```python
from build123d import *

# Parameters (mm, degrees)
SKETCH1_R           = 39.3
BOSS_EXTRUDE1_DEPTH = 21.4
FILLET1_R           = 1.5
SKETCH2_R           = 4
CUT_EXTRUDE1_DEPTH  = 50


with BuildPart() as part:
    # Sketch1 → Boss-Extrude1 (new body)
    with BuildSketch(Plane(origin=(0, 0, 0), x_dir=(1, 0, 0), z_dir=(0, 1, 0))):
        Circle(SKETCH1_R)
    extrude(amount=BOSS_EXTRUDE1_DEPTH)

    # Fillet1
    fillet1_edges = [part.edges().sort_by_distance(p)[0] for p in [
        (-39.3, 21.4, 0),
    ]]
    fillet(fillet1_edges, radius=FILLET1_R)

    # Sketch2 → Cut-Extrude1 (cut)
    with BuildSketch(Plane.XY.offset(39.3)):
        with Locations((-20, 9.95)):
            Circle(SKETCH2_R)
        with Locations((20, 9.95)):
            Circle(SKETCH2_R)
    extrude(amount=-CUT_EXTRUDE1_DEPTH, mode=Mode.SUBTRACT)


solid = part.part
```
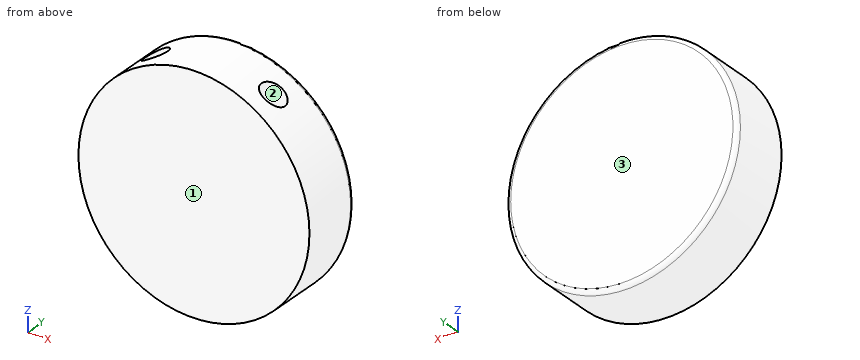
Can you work these out from the model? Positions are in its coordinate system, mm. Face numbers are marked on the shaded views. Coordinates: 2 decimals unless noted, no trailing zeros. Write each loop counter-clockwise with the first axis right and the second up, starting at its lowest first coordinate (ties: lowest second). Pieces come first, ordered by that corner, then holes. Notation, with made-up numbers: M 33,-11 L 77,-11 A14 cw 77,-1 Z; hole C 39.25,-24 d6. An arc over 180 degrees is marked long. Write item = value, one per line. Start each with the question number.
Q1. I'm going to push flat-ended pins straight in: pin 1 (4 mm diameter, centred on y = 8, z = 6, fed in from -X); pin 2 (6 mm diameter, centred on x = -26.5, y = 17.5, fed in from -Z); pin 3 (4 mm diameter, centred on x = -20, y = 10, fed in from +Z). Where does each tip first touch, or does it pass through?
Q2. If we section it at A-A, the plane z = 0: Write out the boundary of the cut face in (x, y).
Q3. If I drill on L1, parallel to Y at x = 20, z = 18; L2, parallel to X at y = 9.95, z = 0.5; L3, parallel to X at y = 9.95, z = 3, over which ranges is the centre line in solid material (lowest first)? Write a range as [from, to].
Q4. If we section it at B-B, the plane y = 17.75: Write out the boundary of the cut face in (x, z).
Q5. If we section it at D-D, the plane y = 9.95: Write out the boundary of the cut face in (x, z), then the cut area to 3 significant figures.
Q6. If we section it at C-C, the plane z = -8: State how many separate pieces and enclosed holes the cut face has, then the cut area to 3 significant figures.
Q7. Thinking about a two-plate mould opening in Y: for the marked faces 1, 2 and 3, which applies, released by +Y, released by -Y, zero draft, split by the parting line, or undercut?
Check sheet entries:
q1.pin_1 = -39.1
q1.pin_2 = -31.5
q1.pin_3 = -10.7
q2.outline = M -39.3,0 L 39.3,0 L 39.3,19.9 A1.5 ccw 37.8,21.4 L -37.8,21.4 A1.5 ccw -39.3,19.9 Z; hole C -20,9.95 d8; hole C 20,9.95 d8
q3.L1 = [0, 5.95], [13.95, 21.4]
q3.L2 = [-39.3, -24], [-16, 16], [24, 39.3]
q3.L3 = [-39.19, -24], [-16, 16], [24, 39.19]
q4.outline = C 0,0 d78.6
q5.outline = M -24,-10.7 L -24,31.12 A39.3 ccw long 24,31.12 L 24,-10.7 L 16,-10.7 L 16,35.9 A39.3 ccw -16,35.9 L -16,-10.7 Z
q5.area = 4,140 mm²
q6.separate_pieces = 1
q6.enclosed_holes = 2
q6.area = 1,550 mm²
q7.face_1 = released by -Y
q7.face_2 = undercut
q7.face_3 = released by +Y
